Answer from the drawing. Dimensions are ordinates in mm from the lowest x, y and z of the part. A direction names the side the tool comes from. Coordinates: 2 decimals unless noted, no trailing zeros. Write each loop counter-clockwise with the first axis right and the second up, starting at its lowest first coordinate (ties: lowest second). Pieces come first, ordered by that corner, then holes. Notation, with made-up numbers: (-5.5, 37) -> (25.5, 37) arc R26 ccw to (25.5, 71) -> close; hole circle Ø2 at (72, -2). An arc over 180 degrees is marked (long way). Answer as a JSON object with one key per item and string values. Group by question number.
(1) Find section D-D (z = 3.5). Give the vertices of the cut face in (x, y).
(2) Find section B-B (y = 35). Give the vertices of the cut face in (x, z).
(3) Find section A-A (z = 8). Give the vertices of the cut face in (x, y).
(4) Straight lines are drawn through the part: L1, parallel to Y at x = 12, z = 2; L2, parallel to Y at x = 14.5, z = 10; L3, parallel to Y at x = 7, z = 8.75 (1 decimal). For each, find the intervals that lie inside material, in ascending order.
(5) For a pull along Y with two mould halves and no side action, classify the marked faces 1, 2, 3 and 4 as +Y half, -Y half, draft (parallel to the pull), parting line (faces both ways), or undercut.
(6) Which of the six approach directions +Z, -Z, +X, -X, +Y, -Y give full straight-line access (tool end or side, diameter ignored) to the marked faces 5 and 6?
(7) A flat-ended cylindrical pin translates along its axis: P1, Ø2, axis at y = 22, z = 10, coming from the -X side. Find the tip coordinate at first contact, or state that the pin passes through.
(8) Find section C-C (x = 11). Give the vertices of the cut face in (y, z).
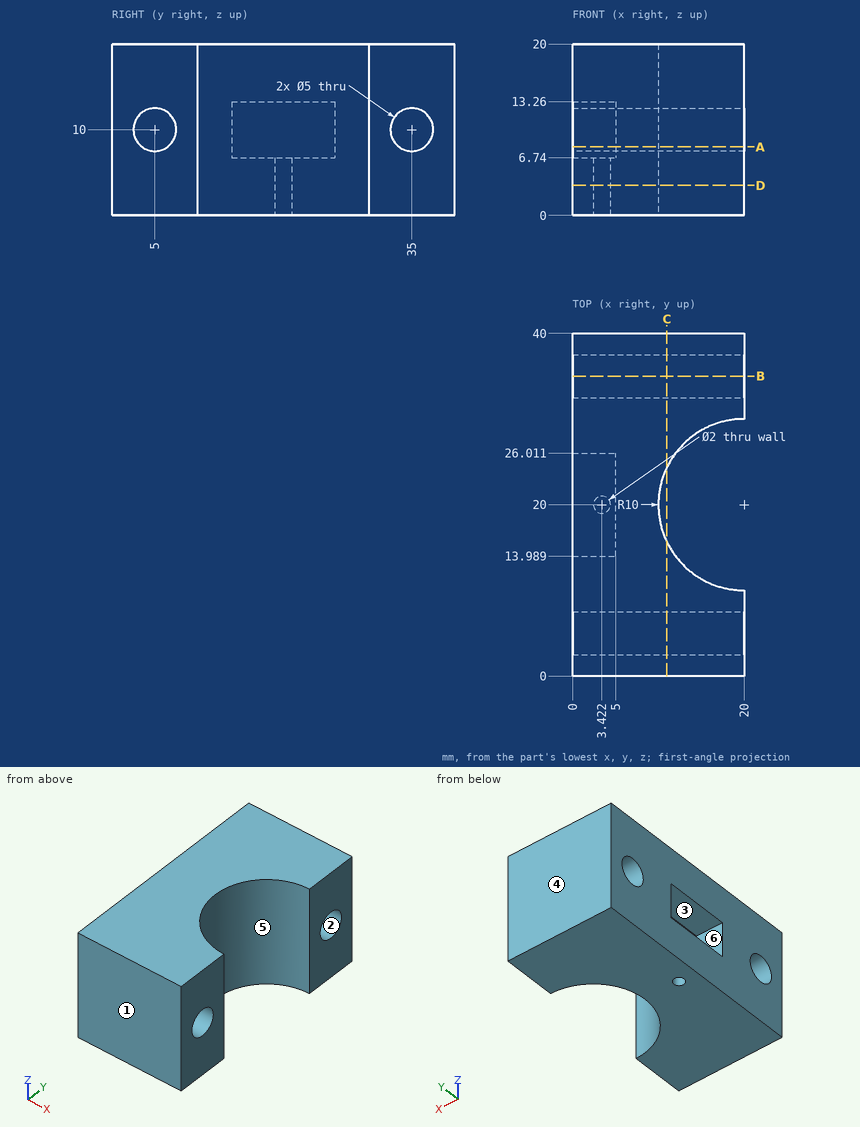
Results below:
{
 "1": {"outline": "(0, 0) -> (20, 0) -> (20, 10) arc R10 cw to (20, 30) -> (20, 40) -> (0, 40) -> close; hole circle Ø2 at (3.42, 20)"},
 "2": {"outline": "(0, 0) -> (20, 0) -> (20, 7.5) -> (0, 7.5) -> close; (0, 12.5) -> (20, 12.5) -> (20, 20) -> (0, 20) -> close"},
 "3": {"outline": "(0, 0) -> (20, 0) -> (20, 3.5) -> (0, 3.5) -> close; (0, 6.5) -> (20, 6.5) -> (20, 10) arc R10 cw to (20, 30) -> (20, 33.5) -> (0, 33.5) -> (0, 26.01) -> (5, 26.01) -> (5, 13.99) -> (0, 13.99) -> close; (0, 36.5) -> (20, 36.5) -> (20, 40) -> (0, 40) -> close"},
 "4": {"L1": "y = 0 to 14, 26 to 40", "L2": "y = 0 to 2.5, 7.5 to 11.65, 28.35 to 32.5, 37.5 to 40", "L3": "y = 0 to 2.8, 7.2 to 32.8, 37.2 to 40"},
 "5": {"face 1": "-Y half", "face 2": "undercut", "face 3": "undercut", "face 4": "+Y half"},
 "6": {"face 5": "+Z, -Z, +X", "face 6": "-X"},
 "7": {"P1": "stops at x = 5"},
 "8": {"outline": "(0, 0) -> (15.64, 0) -> (15.64, 20) -> (0, 20) -> close; (24.36, 0) -> (40, 0) -> (40, 20) -> (24.36, 20) -> close; hole circle Ø5 at (5, 10); hole circle Ø5 at (35, 10)"}
}
